Can you work these out from the drawing? Everything is in mm from the part's minimum corner. A direction names the side the tool comes from. Coordinates: 2 decimals unless noted, no trailing zeros. Order: outer loops, then holes, each group sorted by start corner. A loop starts at its lowest first (then second) coordinate and runs counter-clockwise, first axis right, second up. Notation, with made-up numbers: M 77.5,-31 L 97.5,-31 A32 cw 97.5,1 Z; hole C -22,22.25 d4. An arc over 180 degrees is marked long. Answer as a JSON object with one key per item and string values.
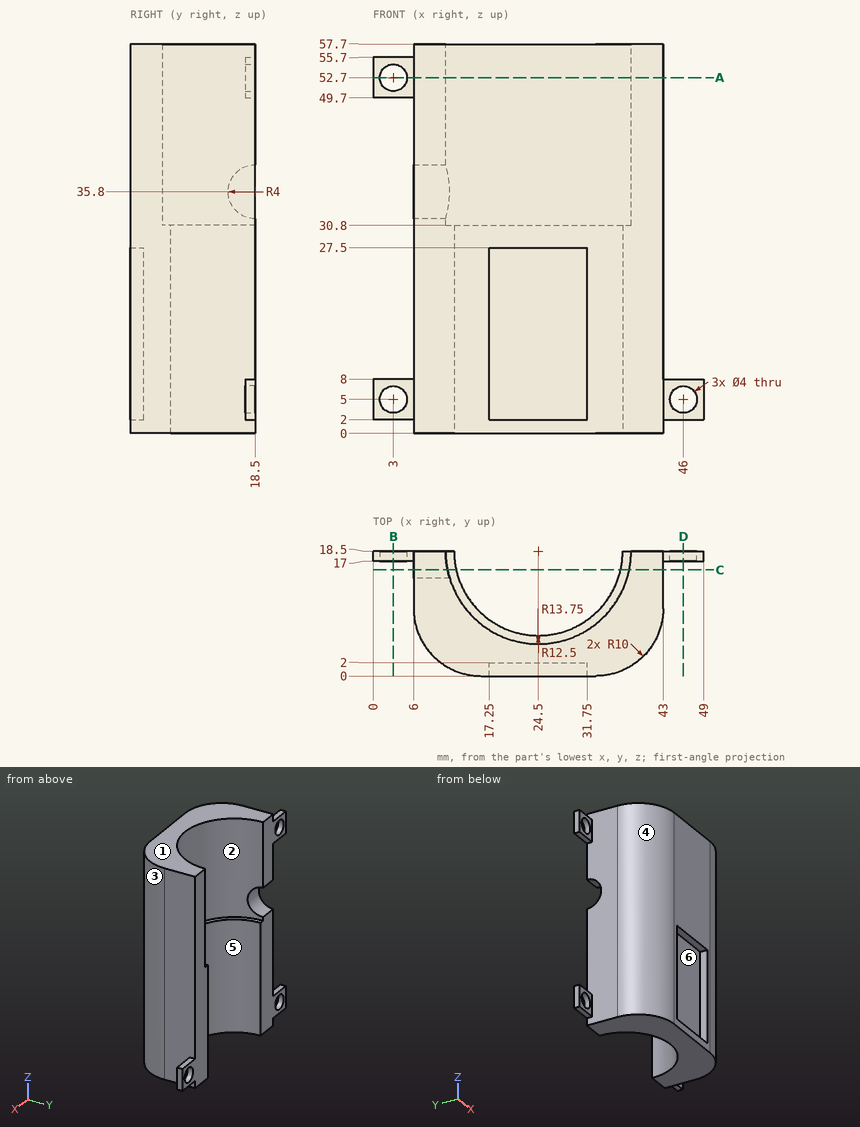
Item 1: Please list where these lines run through material, in increasing order: line 1 (Z direction, x = 3, y = 18.15); line 2 (X direction, y = 18.1, z = 5); line 3 (X direction, y = 17.75, z = 54.5).
Answers follow:
{"line 1": "z = 2 to 3, 7 to 8, 49.7 to 50.7, 54.7 to 55.7", "line 2": "x = 0 to 1, 5 to 12.01, 36.99 to 44, 48 to 49", "line 3": "x = 0 to 2.13, 3.87 to 10.77, 38.23 to 43"}
Item 2: I want a section at C-C, the plane y = 15.75. Write out the boundary of the cut face in (x, z), plus the area to 3 significant figures.
Answers follow:
{"outline": "M 6,0 L 12.31,0 L 12.31,30.8 L 11.03,30.8 L 11.03,32.9 L 6,32.9 Z; M 6,38.7 L 11.03,38.7 L 11.03,57.7 L 6,57.7 Z; M 36.69,0 L 43,0 L 43,57.7 L 37.97,57.7 L 37.97,30.8 L 36.69,30.8 Z", "area": "630 mm^2"}
Item 3: Which directions (+Z, -Z, +X, -X, +Y, -Y) give clear straight access to the entire face, cutting with the end or side of a thin tool? Please do the marked faces 5 and 6.
Answers follow:
{"face 5": "+Z, -Z, +Y", "face 6": "-Y"}
Item 4: I want a section at B-B, the plane x = 3. Write out the boundary of the cut face in (y, z).
Answers follow:
{"outline": "M 17,2 L 18.5,2 L 18.5,3 L 17,3 Z; M 17,7 L 18.5,7 L 18.5,8 L 17,8 Z; M 17,49.7 L 18.5,49.7 L 18.5,50.7 L 17,50.7 Z; M 17,54.7 L 18.5,54.7 L 18.5,55.7 L 17,55.7 Z"}
Item 5: I'm going to push flat-ended pins straight in: pin 1 (1.5 mm diameter, centred on y = 7.5, z = 47.5, fed in from -X); pin 2 (1.6 mm diameter, centred on x = 3, y = 18, fed in from +Z); pin 3 (2.5 mm diameter, centred on x = 46, z = 5, fed in from +Y); pin 4 (0.6 mm diameter, centred on y = 1.5, z = 20, fed in from +X). Where does each tip first touch, or does it pass through?
Answers follow:
{"pin 1": "stops at x = 6.15", "pin 2": "stops at z = 55.7", "pin 3": "passes through", "pin 4": "stops at x = 38.72"}
Item 6: I want a section at A-A, the plane z = 52.7. Write out the boundary of the cut face in (x, y), plus the area to 3 significant figures.
Answers follow:
{"outline": "M 0,17 L 1,17 L 1,18.5 L 0,18.5 Z; M 5,17 L 6,17 L 6,10 A10 ccw 16,0 L 33,0 A10 ccw 43,10 L 43,18.5 L 38.25,18.5 A13.75 cw 10.75,18.5 L 5,18.5 Z", "area": "348 mm^2"}
Item 7: I want a section at D-D, the plane x = 46. Write out the boundary of the cut face in (y, z), plus the area to 3 significant figures.
Answers follow:
{"outline": "M 17,2 L 18.5,2 L 18.5,3 L 17,3 Z; M 17,7 L 18.5,7 L 18.5,8 L 17,8 Z", "area": "3.00 mm^2"}
Item 8: If we mould it in two halves opening along X, with no side actions, what happens to the marked faces 1, 2, 3 and 4? For each: pulls with the +X half, pulls with the -X half, needs draft (parallel to the pull), parting line crosses it, or undercut.
Answers follow:
{"face 1": "needs draft", "face 2": "undercut", "face 3": "pulls with the +X half", "face 4": "pulls with the -X half"}
